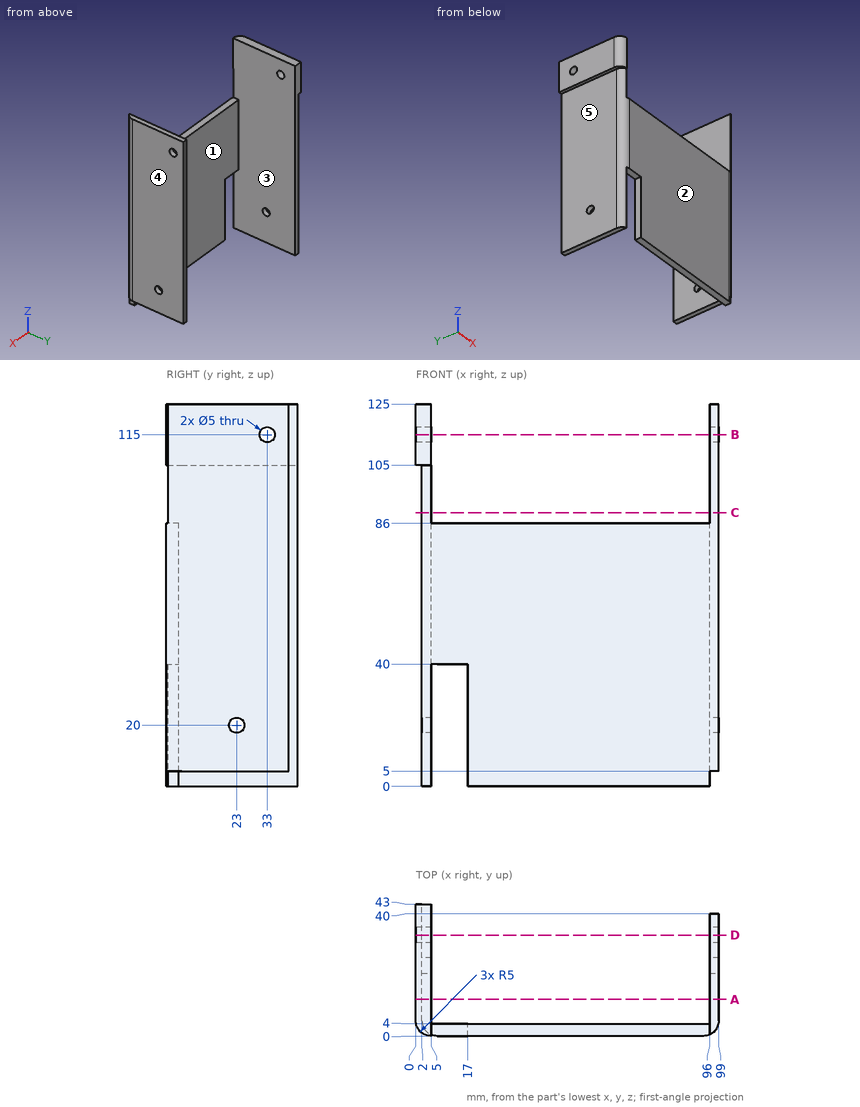
Drawing for the job (mm, zero at the part's lowest x, y, z). A direction names the side the tool comes from. Coordinates: 2 decimals unless noted, no trailing zeros. Write each loop counter-clockwise with the first axis right and the second up, starting at its lowest first coordinate (ties: lowest second). Pieces come first, ordered by that corner, then holes. Notation, with made-up numbers: (-37, 25.25) -> (-2, 25.25) arc R28 ccw to (-2, 60.25) -> close; hole circle Ø8 at (-1, 25). An arc over 180 degrees is marked (long way). One line per item, written item: value. Start each with the question number.
1) Probe probe 1 along Z at (x, y) = (3.9, 23); probe 2 along X at (y, z) = (10, 112.5); probe 3 along X at (y, z) = (21.5, 68.5). List the from-to ranges inside material, lowest first.
2) Which spindle directions (+Z, -Z, +X, -X, +Y, -Y) get a long thin tool onto all of the face, cutting with end or side? Do the marked faces 1 and 2. Say none if no direction does.
3) Slice it at A-A on y = 12. Write the cut outline in (x, z), then the cut area to 3 significant figures.
4) Pull direction X, two halves, no side cores. Call the marked faces 3, 4 and 5: +X half, -X half, draft (parallel to the pull), parting line (faces both ways), or undercut.
5) Slice it at C-C on z = 89.5. Write the cut outline in (x, y), then the cut area to 3 significant figures.
6) Slice it at B-B on z = 115. Count the separate pieces of the cut face and the enclosed holes in it, then the cut area to 3 significant figures.
7) Slice it at D-D on y = 33. Write the cut outline in (x, z), then the cut area to 3 significant figures.
8) Flat gauge pins, fed straight in: pin 1 Ø19 at (y, z) = (32.5, 32.5) entering from -X; pin 2 Ø1.2 at (x, y) = (41, 2.5) entering from +Z; pin 3 Ø3 at (x, z) = (17, 41.5) entering from +Y. Where does each tip first touch, or does it go through?
Answers follow:
1. probe 1: 0 to 17.5, 22.5 to 125
1. probe 2: 0 to 5, 96 to 99
1. probe 3: 2 to 5, 96 to 99
2. face 1: +Z, -Z, +Y
2. face 2: +Z, -Z, +X, -X, -Y
3. outline: (0, 105) -> (2, 105) -> (2, 0) -> (5, 0) -> (5, 125) -> (0, 125) -> close; (96, 5) -> (99, 5) -> (99, 125) -> (96, 125) -> close
3. area: 775 mm2
4. face 3: undercut
4. face 4: +X half
4. face 5: -X half
5. outline: (2, 5) arc R5 ccw to (5, 0.42) -> (5, 43) -> (2, 43) -> close; (96, 0.42) arc R5 ccw to (99, 5) -> (99, 40) -> (96, 40) -> close
5. area: 239 mm2
6. separate pieces: 4
6. enclosed holes: 0
6. area: 285 mm2
7. outline: (0, 105) -> (2, 105) -> (2, 0) -> (5, 0) -> (5, 112.5) -> (0, 112.5) -> close; (0, 117.5) -> (5, 117.5) -> (5, 125) -> (0, 125) -> close; (96, 5) -> (99, 5) -> (99, 112.5) -> (96, 112.5) -> close; (96, 117.5) -> (99, 117.5) -> (99, 125) -> (96, 125) -> close
7. area: 735 mm2
8. pin 1: x = 2
8. pin 2: z = 86
8. pin 3: y = 4
